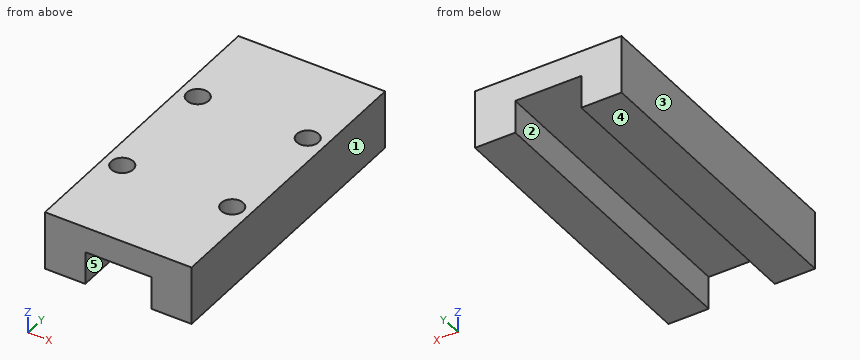
from build123d import *

# Parameters (mm, degrees)
F0_W     = 20
F0_H     = 8
F1_DEPTH = 20.5
F2_W     = 9
F2_H     = 4.5
F3_DEPTH = 41.001
F4_R     = 1.5
F5_DEPTH = 5


with BuildPart() as f1:
    # F0 (on Front) → F1 (new body, symmetric)
    with BuildSketch(Plane.XZ):
        Rectangle(F0_W, F0_H)
    extrude(amount=F1_DEPTH, both=True)

    # F2 (on face) → F3 (cut, through all)
    with BuildSketch(Plane.XZ.offset(20.5)):
        with Locations((0, -1.75)):
            Rectangle(F2_W, F2_H)
    extrude(amount=-F3_DEPTH, mode=Mode.SUBTRACT)

    # F4 (on face) → F5 (cut)
    with BuildSketch(Plane.XY.offset(4)):
        with Locations((-7.5, 8)):
            Circle(F4_R)
        with Locations((7.5, 8)):
            Circle(F4_R)
        with Locations((7.5, -8)):
            Circle(F4_R)
        with Locations((-7.5, -8)):
            Circle(F4_R)
    extrude(amount=-F5_DEPTH, mode=Mode.SUBTRACT)


solid = f1.part
Part model, mm, in its own coordinate system. Face numbers are marked on the shaded views. A direction names the side the tool comes from. Round coordinates to 2 decimals unless told otherwise and drop trailing zeros. Write each loop counter-clockwise with the first axis right and the second up, starting at its lowest first coordinate (ties: lowest second). Pieces come first, ordered by that corner, then holes. Notation, with made-up numbers: M -33,26.25 L 21,26.25 A26 cw 21,44.25 Z; hole C -37.5,5 d9. An arc over 180 degrees is marked long. Return JSON: item names as keys, results as strings. Group by question number.
(1) Saw through at B-B on y = 4.5. Write the cut outline in (x, z).
(2) Saw through at A-A on z = -2. Write the cut outline in (x, y), then the cut area to 3 significant figures.
(3) Saw through at C-C on z = 1.75. Write the cut outline in (x, y), then the cut area to 3 significant figures.
(4) Pin check, flat tip, straight feed: pin 1 Ø1.5 at (x, y) = (7.5, 8) entering from +Z. Stop position of the tip, or through.
(5) Which spindle directions (+Z, -Z, +X, -X, +Y, -Y) get a long thin tool onto all of the face, cutting with end or side? Do the marked faces 1 and 2. Say none if no direction does.
(6) Two-plate mould, pull along X, no slides. Class the marked faces 3, 4 and 5: +X half, -X half, draft (parallel to the pull), parting line (faces both ways), or undercut.
(7) Saw through at D-D on x = 6.5. Write the cut outline in (y, z), then the cut area to 3 significant figures.
(8) Drill centre lines: probe 1 along Y at (x, z) = (-7.5, 0.3); probe 2 along X at (y, z) = (-16.5, -1); probe 3 along X at (y, z) = (8.5, -0.75). Where is each one in solid material? Low to high.
Returned:
{
 "1": {"outline": "M -10,-4 L -4.5,-4 L -4.5,0.5 L 4.5,0.5 L 4.5,-4 L 10,-4 L 10,4 L -10,4 Z"},
 "2": {"outline": "M -10,-20.5 L -4.5,-20.5 L -4.5,20.5 L -10,20.5 Z; M 4.5,-20.5 L 10,-20.5 L 10,20.5 L 4.5,20.5 Z", "area": "451 mm²"},
 "3": {"outline": "M -10,-20.5 L 10,-20.5 L 10,20.5 L -10,20.5 Z; hole C -7.5,-8 d3; hole C -7.5,8 d3; hole C 7.5,-8 d3; hole C 7.5,8 d3", "area": "792 mm²"},
 "4": {"pin 1": "z = -1"},
 "5": {"face 1": "+Z, -Z, +X, +Y, -Y", "face 2": "-Z, +Y, -Y"},
 "6": {"face 3": "-X half", "face 4": "draft", "face 5": "undercut"},
 "7": {"outline": "M -20.5,-4 L 20.5,-4 L 20.5,4 L 9.12,4 L 9.12,-1 L 6.88,-1 L 6.88,4 L -6.88,4 L -6.88,-1 L -9.12,-1 L -9.12,4 L -20.5,4 Z", "area": "306 mm²"},
 "8": {"probe 1": "-20.5 to -9.5, -6.5 to 6.5, 9.5 to 20.5", "probe 2": "-10 to -4.5, 4.5 to 10", "probe 3": "-10 to -8.91, -6.09 to -4.5, 4.5 to 6.09, 8.91 to 10"}
}
